```python
from build123d import *

# Parameters (mm, degrees)
SKETCH1_R                   = 1.5
BOSS_EXTRUDE1_DEPTH         = 5
TAP_DRILL_FOR_M3_TAP1_D     = 2.5
TAP_DRILL_FOR_M3_TAP2_D     = 2.5
TAP_DRILL_FOR_M3_TAP2_DEPTH = 4
TAP_DRILL_FOR_M3_TAP2_TIP   = 0.751075774
FILLET1_R                   = 1


with BuildPart() as part:
    # Sketch1 → Boss-Extrude1 (new body)
    with BuildSketch(Plane.XY):
        with BuildLine():
            Line((-10, 25), (-2, 25))
            ThreePointArc((-2, 25), (1.221825407, 17.221825407), (9, 14))
            Line((9, 14), (10, 14))
            Line((10, 14), (10, 0.5))
            Line((10, 0.5), (10, 0))
            Line((10, 0), (-10, 0))
            Line((-10, 0), (-14.5, 0))
            Line((-14.5, 0), (-14.5, 25))
            Line((-14.5, 25), (-10, 25))
        make_face()
        with Locations((-7.5, 17)):
            Circle(SKETCH1_R, mode=Mode.SUBTRACT)
    extrude(amount=BOSS_EXTRUDE1_DEPTH)

    # Tap Drill for M3 Tap1 (through all)
    with Locations(Plane.XY.offset(5)):
        with Locations((-7, 13), (-7, 21), (5, 10), (0.5, 3.5), (7.5, 3.5)):
            Hole(TAP_DRILL_FOR_M3_TAP1_D / 2)

    # Tap Drill for M3 Tap2
    with Locations(Plane(origin=(0, 0, 0), x_dir=(-1, 0, 0), z_dir=(0, -1, 0))):
        with Locations((3.75, -2.5), (10.25, -2.5)):
            Hole(TAP_DRILL_FOR_M3_TAP2_D / 2, depth=TAP_DRILL_FOR_M3_TAP2_DEPTH)
            with Locations((0, 0, -(TAP_DRILL_FOR_M3_TAP2_DEPTH + TAP_DRILL_FOR_M3_TAP2_TIP / 2))):  # 118° drill point
                Cone(0, TAP_DRILL_FOR_M3_TAP2_D / 2, TAP_DRILL_FOR_M3_TAP2_TIP, mode=Mode.SUBTRACT)

    # Fillet1
    fillet1_edges = [part.edges().sort_by_distance(p)[0] for p in [
        (-14.5, 25, 2.5),
        (-2, 25, 2.5),
        (10, 14, 2.5),
    ]]
    fillet(fillet1_edges, radius=FILLET1_R - 0.0001)  # a hair under: the kernel refuses the full size


solid = part.part
```
Check sheet for the modelled part. Datum: model origin and axes. Units: mm. A direction names the side the tool comes from. Coordinates: 2 decimals unless noted, no trailing zeros. Order: outer loops, then holes, each group sorted by start corner. A loop starts at its lowest first (then second) coordinate and runs counter-clockwise, first axis right, second up. Notation, with made-up numbers: M 38,-11 L 50,-11 A27 ccw 50,8 Z; hole C 42.5,-37 d4. An arc over 180 degrees is marked long. Write each question's results on one line, items separated by ' | '. Start each with the question number.
1. Cross-section at B-B on z = 0.95. State how many separate pieces and enclosed holes the cut face has, and give its area (3 significant figures).
2. Cross-section at C-C on x = 7.5. Record the cut outline in (y, z), and give its area (3 significant figures).
3. Access from +Z, -Z, +X, -X, +Y, -Y to the whole of each face (thin tool, end or side, straight path). Record for faces 1 (the face through (-2.274, 24.729, 2.535)), 2 (the face through (-4.671, 2.028, 1.655)).
4. Material ranges on probe 1 along X at (y, z) = (2, 2.8); probe 2 along Y at (x, z) = (-7.5, 1.15); probe 3 along X at (y, z) = (2, 3.55), recorded low to high.
5. Go/stop test with a flat-tipped pin: P1, Ø3, axis at x = -10.25, z = 2.5, coming from the -Y side. Record where the tip stops, or that it passes through.
6. Mould release check, pull along X, two halves, no side actions. Record for faces 3 (the face through (-6.73, 19.78, 2.46)), 4 (the face through (-2, 0, 2)), 5 (the face through (9.699, 13.715, 2.535)), 6 (the face through (-14.199, 24.715, 2.535)): +X half, -X half, draft (parallel to the pull), parting line (faces both ways), or undercut.
7. Cross-section at A-A on y = 10. Record the cut outline in (x, z), and give its area (3 significant figures).
8. Cross-section at D-D on x = -7. Record the cut outline in (y, z).
Checks:
1) separate pieces: 1 | enclosed holes: 6 | area: 474 mm²
2) outline: M 0,0 L 2.25,0 L 2.25,5 L 0,5 Z; M 4.75,0 L 14.1,0 L 14.1,5 L 4.75,5 Z | area: 58.0 mm²
3) face 1: +Z, -Z, +X, +Y | face 2: -Y
4) probe 1: x = -14.5 to -11.46, -9.04 to -4.96, -2.54 to 10 | probe 2: y = 0 to 11.85, 14.15 to 15.5, 18.5 to 19.85, 22.15 to 25 | probe 3: x = -14.5 to -10.93, -9.57 to -4.43, -3.07 to 10
5) P1: stops at y = 0
6) face 3: undercut | face 4: draft | face 5: +X half | face 6: -X half
7) outline: M -14.5,0 L 3.75,0 L 3.75,5 L -14.5,5 Z; M 6.25,0 L 10,0 L 10,5 L 6.25,5 Z | area: 110 mm²
8) outline: M 0,0 L 11.75,0 L 11.75,5 L 0,5 Z; M 14.25,0 L 15.59,0 L 15.59,5 L 14.25,5 Z; M 18.41,0 L 19.75,0 L 19.75,5 L 18.41,5 Z; M 22.25,0 L 25,0 L 25,5 L 22.25,5 Z
